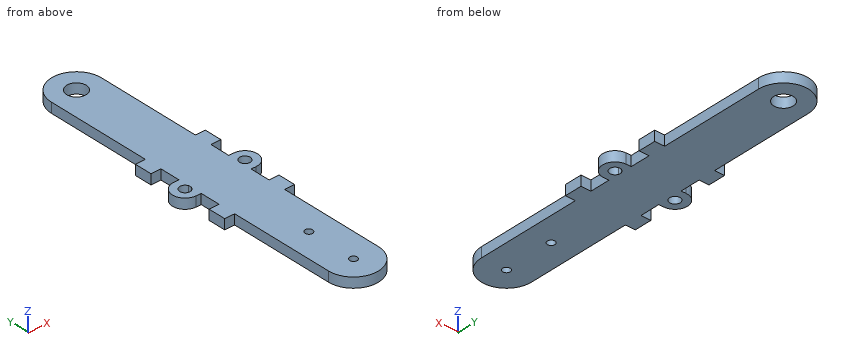
```python
from build123d import *

# Parameters (mm, degrees)
ESQUISSE1_W             = 20
ESQUISSE1_H             = 144
ESQUISSE1_R             = 1.5
ESQUISSE1_R_2           = 3.9
BOSS_EXTRU_1_DEPTH      = 4
CONG_1_RADIUS           = 10
CONG_1_LENGTH           = 4
ESQUISSE2_W             = 4
ESQUISSE2_H             = 7
BOSS_EXTRU_2_DEPTH      = 4
ESQUISSE3_R             = 1.5
ENL_V_MAT_EXTRU_1_DEPTH = 75.087785768
CONG_2_RADIUS           = 10
CONG_2_LENGTH           = 4
ESQUISSE4_R             = 2.1
ENL_V_MAT_EXTRU_2_DEPTH = 75.087785768


with BuildPart() as part:
    # Esquisse1 → Boss.-Extru.1 (new body)
    with BuildSketch(Plane.XY):
        Rectangle(ESQUISSE1_W, ESQUISSE1_H)
        with Locations((0, -62)):
            Circle(ESQUISSE1_R, mode=Mode.SUBTRACT)
        with Locations((0, 62)):
            Circle(ESQUISSE1_R_2, mode=Mode.SUBTRACT)
    extrude(amount=BOSS_EXTRU_1_DEPTH)

    # Congé1: full round fillet: the end face becomes a half cylinder, R = half its width
    cong_1_face = Plane((0, 72, 2), x_dir=(0, 0, 1), z_dir=(0, 1, 0))  # on the end face: x along it, z out of the body
    cong_1_slab = cong_1_face.offset(-CONG_1_RADIUS / 2) * Box(CONG_1_LENGTH, 2 * CONG_1_RADIUS, CONG_1_RADIUS, mode=Mode.PRIVATE)  # the body's end, R deep
    cong_1_round = Plane((0, 62, 2), x_dir=(0, 1, 0), z_dir=(0, 0, 1)) * Cylinder(CONG_1_RADIUS, CONG_1_LENGTH, mode=Mode.PRIVATE)  # its axis R under the face
    add(cong_1_slab - cong_1_round, mode=Mode.SUBTRACT)

    # Esquisse2 → Boss.-Extru.2 (add)
    with BuildSketch(Plane.XY.offset(4)):
        with BuildLine():
            Line((-10, 0.640312424), (-10, 5))
            Line((-10, 5), (-12, 5))
            ThreePointArc((-12, 5), (-17, 0), (-12, -5))
            Line((-12, -5), (-10, -5))
            Line((-10, -5), (-10, -0.640312424))
            ThreePointArc((-10, -0.640312424), (-14.1, 0), (-10, 0.640312424))
        make_face()
        with Locations((-12, 16.5)):
            Rectangle(ESQUISSE2_W, ESQUISSE2_H)
        with Locations((-12, -16.5)):
            Rectangle(ESQUISSE2_W, ESQUISSE2_H)
    boss_extru_2 = extrude(amount=-BOSS_EXTRU_2_DEPTH)

    # Esquisse3 → Enlèv. mat.-Extru.1 (cut, through all)
    with BuildSketch(Plane(origin=(0, 0, 0), x_dir=(-1, 0, 0), z_dir=(0, 0, -1))):
        with Locations((0, -42)):
            Circle(ESQUISSE3_R)
    extrude(amount=-ENL_V_MAT_EXTRU_1_DEPTH, mode=Mode.SUBTRACT)

    # Congé2: full round fillet: the end face becomes a half cylinder, R = half its width
    cong_2_face = Plane((0, -72, 2), x_dir=(0, 0, 1), z_dir=(0, -1, 0))  # on the end face: x along it, z out of the body
    cong_2_slab = cong_2_face.offset(-CONG_2_RADIUS / 2) * Box(CONG_2_LENGTH, 2 * CONG_2_RADIUS, CONG_2_RADIUS, mode=Mode.PRIVATE)  # the body's end, R deep
    cong_2_round = Plane((0, -62, 2), x_dir=(0, -1, 0), z_dir=(0, 0, 1)) * Cylinder(CONG_2_RADIUS, CONG_2_LENGTH, mode=Mode.PRIVATE)  # its axis R under the face
    add(cong_2_slab - cong_2_round, mode=Mode.SUBTRACT)

    # Esquisse4 → Enlèv. mat.-Extru.2 (cut, through all)
    with BuildSketch(Plane.XY.offset(4)):
        with Locations((-12, 0)):
            Circle(ESQUISSE4_R)
    enl_v_mat_extru_2 = extrude(amount=-ENL_V_MAT_EXTRU_2_DEPTH, mode=Mode.SUBTRACT)

    # Symétrie1: Boss.-Extru.2, Enlèv. mat.-Extru.2 across plane
    add(boss_extru_2.mirror(Plane(origin=(0, 0, 0), x_dir=(0, 0, 1), z_dir=(1, 0, 0))))
    add(enl_v_mat_extru_2.mirror(Plane(origin=(0, 0, 0), x_dir=(0, 0, 1), z_dir=(1, 0, 0))), mode=Mode.SUBTRACT)


solid = part.part
```
Geometry check sheet. Reference: the model listing, model coordinates, mm. Give positions to 0.01 mm unless a question says otherwise; leave off trailing zeros. Loops run counter-clockwise (first coordinate to the right, second up) from the corner with the lowest first, then second, coordinate; pieces in that order, holes last. Notation, with made-up numbers: (-2.5, -18.75) - (36.5, -18.75) arc R20 cw to (36.5, -4.75) - close; hole circle Ø7 at (-14, 54.5). An arc over 180 degrees is marked (long way). Use CSV: the item, a comma, the result in double quotes. Start each with the question number.
Q1. Section check C-C, the plane x = -6. Record the cut outline in (y, z).
Q2. Section check A-A, the plane x = 0. Record the cut outline in (y, z).
Q3. Section check B-B, the plane z = 1.5. Count the separate pieces of the cut face and the enclosed holes in it, and give its area (3 significant figures).
Q4. Section check D-D, the plane y = -31.5. Record the cut outline in (x, z), and give its area (3 significant figures).
Q5. Go/stop test with flat-tipped pins: pin 1 Ø2 at (y, z) = (33, 2) entering from -X; pin 2 Ø1.2 at (x, z) = (-11, 2.5) entering from -Y; pin 3 Ø1 at (y, z) = (-3, 2) entering from +X. Record where each tip stops, or that it passes through.
Q6. Scan lines: probe 1 along Y at (x, z) = (0, 1.9); probe 2 along Y at (x, z) = (-12, 2.1); probe 3 along X at (y, z) = (-59, 0.25). Record each from-to range of solid material in increasing order. Write a range as from..to.
Findings below:
1,outline,"(-70, 0) - (70, 0) - (70, 4) - (-70, 4) - close"
2,outline,"(-72, 0) - (-63.5, 0) - (-63.5, 4) - (-72, 4) - close; (-60.5, 0) - (-43.5, 0) - (-43.5, 4) - (-60.5, 4) - close; (-40.5, 0) - (58.1, 0) - (58.1, 4) - (-40.5, 4) - close; (65.9, 0) - (72, 0) - (72, 4) - (65.9, 4) - close"
3,separate pieces,"1"
3,enclosed holes,"5"
3,area,"2,940 mm^2"
4,outline,"(-10, 0) - (10, 0) - (10, 4) - (-10, 4) - close"
4,area,"80.0 mm^2"
5,pin 1,"stops at x = -10"
5,pin 2,"stops at y = -20"
5,pin 3,"stops at x = 16.33"
6,probe 1,"y = -72..-63.5, -60.5..-43.5, -40.5..58.1, 65.9..72"
6,probe 2,"y = -20..-13, -5..-2.1, 2.1..5, 13..20"
6,probe 3,"x = -10..10"
